from build123d import *

# Parameters (mm, degrees)
BOSS_EXTRUDE1_DEPTH = 15


with BuildPart() as part:
    # Sketch3 → Boss-Extrude1 (new, symmetric)
    with BuildSketch(Plane(origin=(0, 0, 0), x_dir=(1, 0, 0), z_dir=(0, 1, 0))):
        with BuildLine():
            Line((-5.617617549, 4.318), (5.617617549, 4.318))
            Line((5.617617549, 4.318), (9.385342517, 4.318))
            ThreePointArc((9.385342517, 4.318), (9.843335579, 4.507706938), (10.033042517, 4.9657))
            Line((10.033042517, 4.9657), (10.033042517, 5.533957912))
            ThreePointArc((10.033042517, 5.533957912), (9.983739138, 5.781822339), (9.843335016, 5.991951537))
            Line((9.843335016, 5.991951537), (5.112460341, 10.722814576))
            ThreePointArc((5.112460341, 10.722814576), (3.653919205, 11.69737866), (1.933453584, 12.0396))
            Line((1.933453584, 12.0396), (-1.933453584, 12.0396))
            ThreePointArc((-1.933453584, 12.0396), (-3.653919205, 11.69737866), (-5.112460341, 10.722814576))
            Line((-5.112460341, 10.722814576), (-9.843335016, 5.991951537))
            ThreePointArc((-9.843335016, 5.991951537), (-9.983739138, 5.781822339), (-10.033042517, 5.533957912))
            Line((-10.033042517, 5.533957912), (-10.033042517, 4.9657))
            ThreePointArc((-10.033042517, 4.9657), (-9.843335579, 4.507706938), (-9.385342517, 4.318))
            Line((-9.385342517, 4.318), (-5.617617549, 4.318))
        make_face()
    extrude(amount=BOSS_EXTRUDE1_DEPTH, both=True)


solid = part.part
The listing builds one solid part. Answer for the finished solid, in the listing's coordinates (mm). Give positions to 0.01 mm unless a question says otherwise; leave off trailing zeros. Loops run counter-clockwise (first coordinate to the right, second up) from the corner with the lowest first, then second, coordinate; pieces in that order, holes last. Notation, with made-up numbers: (-26.5, 22.5) - (-17.5, 22.5) arc R20 ccw to (-17.5, 44.5) - close; hole circle Ø7 at (1.25, 20.5). An arc over 180 degrees is marked (long way). Use one line per item in the form item = value.
1. Given pin 1 Ø1 at (x, y) = (8, 2) entering from -Z, flat-ended and moving along its own axis, determine where the tip first touches the part or whether it passes through.
Calculated:
pin_1 = -8.34
2. Section C-C on z = -9.75 is taken. Give the vertices of the cut face in (x, y), then the cut area to 3 significant figures.
Calculated:
outline = (-6.09, -15) - (6.09, -15) - (6.09, 15) - (-6.09, 15) - close
area = 365 mm^2
3. Find the intervals of material crossed by line 1 along X through (y, z) = (-7, -10.75); line 2 along Z through (x, y) = (3.5, -8); line 3 along X through (y, z) = (-2, -8), in increasing order. Write a range as [from, to].
Calculated:
line_1 = [-5.09, 5.09]
line_2 = [-11.76, -4.32]
line_3 = [-7.84, 7.84]
4. Section B-B on x = 6.5 is taken. Give the vertices of the cut face in (y, z), then the cut area to 3 significant figures.
Calculated:
outline = (-15, -9.34) - (15, -9.34) - (15, -4.32) - (-15, -4.32) - close
area = 151 mm^2
5. Section A-A on y = 1.75 is taken. Give the vertices of the cut face in (x, z).
Calculated:
outline = (-10.03, -5.53) arc R0.65 ccw to (-9.84, -5.99) - (-5.11, -10.72) arc R4.5 ccw to (-1.93, -12.04) - (1.93, -12.04) arc R4.5 ccw to (5.11, -10.72) - (9.84, -5.99) arc R0.65 ccw to (10.03, -5.53) - (10.03, -4.97) arc R0.65 ccw to (9.39, -4.32) - (-9.39, -4.32) arc R0.65 ccw to (-10.03, -4.97) - close
